Geometry check sheet. Reference: the model listing, model coordinates, mm. A direction names the side the tool comes from. Coordinates: 2 decimals unless noted, no trailing zeros. Loops run counter-clockwise (first coordinate to the right, second up) from the corner with the lowest first, then second, coordinate; pieces in that order, holes last.
from build123d import *

# Parameters (mm, degrees)
F0_W          = 90
F0_H          = 32
F1_DEPTH      = 65.2
F3_DEPTH      = 25
F4_W          = 90
F4_H          = 65.2
F5_DEPTH      = 32.001
F6_DEPTH      = 62.5
F8_DEPTH      = 16.25
F8_DEPTH_BACK = 78.75
F9_R          = 2
F11_DEPTH     = 78.751


with BuildPart() as f1:
    # F0 (on Front) → F1 (new body)
    with BuildSketch(Plane.XZ):
        with Locations((-2.4301670492, -5.0586230417)):
            Rectangle(F0_W, F0_H)
    extrude(amount=F1_DEPTH)

    # F2 (on face) → F3 (join)
    with BuildSketch(Plane.XZ.offset(65.2)):
        with BuildLine():
            Line((40.5698329508, 10.9413769583), (-45.4301670492, 10.9413769583))
            ThreePointArc((-45.4301670492, 10.9413769583), (-46.8443806115, 10.3555905207), (-47.4301670492, 8.9413769583))
            Line((-47.4301670492, 8.9413769583), (-47.4301670492, 2.9413769583))
            ThreePointArc((-47.4301670492, 2.9413769583), (-46.8443806115, 1.5271633959), (-45.4301670492, 0.9413769583))
            Line((-45.4301670492, 0.9413769583), (-42.2728696535, 0.9413769583))
            ThreePointArc((-42.2728696535, 0.9413769583), (-41.1580897163, 0.6018785968), (-40.4217757411, -0.3013573503))
            Line((-40.4217757411, -0.3013573503), (-32.4385583572, -19.8158887331))
            ThreePointArc((-32.4385583572, -19.8158887331), (-31.7022443821, -20.7191246802), (-30.5874644448, -21.0586230417))
            Line((-30.5874644448, -21.0586230417), (25.7271303465, -21.0586230417))
            ThreePointArc((25.7271303465, -21.0586230417), (26.8419102837, -20.7191246802), (27.5782242589, -19.8158887331))
            Line((27.5782242589, -19.8158887331), (35.5614416428, -0.3013573503))
            ThreePointArc((35.5614416428, -0.3013573503), (36.2977556179, 0.6018785968), (37.4125355552, 0.9413769583))
            Line((37.4125355552, 0.9413769583), (40.5698329508, 0.9413769583))
            ThreePointArc((40.5698329508, 0.9413769583), (41.9840465132, 1.5271633959), (42.5698329508, 2.9413769583))
            Line((42.5698329508, 2.9413769583), (42.5698329508, 8.9413769583))
            ThreePointArc((42.5698329508, 8.9413769583), (41.9840465132, 10.3555905207), (40.5698329508, 10.9413769583))
        make_face()
    extrude(amount=F3_DEPTH)

    # F4 (on face) → F5 (cut, through all)
    with BuildSketch(Plane.XY.offset(10.9413769583)):
        with Locations((-2.4301670492, -32.6)):
            Rectangle(F4_W, F4_H)
    extrude(amount=-F5_DEPTH, mode=Mode.SUBTRACT)

    # F6 (add): a face of the model
    f6_faces = [f1.faces().sort_by_distance(p)[0] for p in [
        (-2.4301670492, -90.2, -3.7537517767),
    ]]
    extrude(f6_faces, amount=-F6_DEPTH)

    # F7 (on face) → F8 (join, two sides)
    with BuildSketch(Plane.XZ.offset(90.2)) as f8_sk:
        with BuildLine():
            Line((21.5698329508, 10.9413769583), (-26.4301670492, 10.9413769583))
            ThreePointArc((-26.4301670492, 10.9413769583), (-27.8443806115, 10.3555905207), (-28.4301670492, 8.9413769583))
            Line((-28.4301670492, 8.9413769583), (-28.4301670492, -19.0586230417))
            ThreePointArc((-28.4301670492, -19.0586230417), (-27.8443806115, -20.4728366041), (-26.4301670492, -21.0586230417))
            Line((-26.4301670492, -21.0586230417), (-16.4301670492, -21.0586230417))
            Line((-16.4301670492, -21.0586230417), (-16.4301670492, -9.1799433853))
            Line((-16.4301670492, -9.1799433853), (-14.3088467056, -7.0586230417))
            Line((-14.3088467056, -7.0586230417), (9.4485126073, -7.0586230417))
            Line((9.4485126073, -7.0586230417), (11.5698329508, -9.1799433853))
            Line((11.5698329508, -9.1799433853), (11.5698329508, -21.0586230417))
            Line((11.5698329508, -21.0586230417), (21.5698329508, -21.0586230417))
            ThreePointArc((21.5698329508, -21.0586230417), (22.9840465132, -20.4728366041), (23.5698329508, -19.0586230417))
            Line((23.5698329508, -19.0586230417), (23.5698329508, 8.9413769583))
            ThreePointArc((23.5698329508, 8.9413769583), (22.9840465132, 10.3555905207), (21.5698329508, 10.9413769583))
        make_face()
    extrude(amount=F8_DEPTH)
    extrude(f8_sk.sketch, amount=-F8_DEPTH_BACK)

    # F9
    f9_edges = [f1.edges().sort_by_distance(p)[0] for p in [
        (-28.430167, -106.45, -5.058623),
        (-2.430167, -11.45, 10.941377),
    ]]
    fillet(f9_edges, radius=F9_R)

    # F10 (on face) → F11 (cut, through all)
    with BuildSketch(Plane.XZ.offset(90.2)):
        Polygon((-16.4301670492, -9.1799433853), (-16.4301670492, -21.0586230417), (11.5698329508, -21.0586230417), (11.5698329508, -9.1799433853), (9.4485126073, -7.0586230417), (-14.3088467056, -7.0586230417), align=None)
    extrude(amount=-F11_DEPTH, mode=Mode.SUBTRACT)


solid = f1.part
(1) Gauge pin test, flat ends, axial feed: pin 1 Ø5 at (x, z) = (-38, 3.5) entering from +Y; pin 2 Ø7 at (y, z) = (-22, 0.5) entering from -X; pin 3 Ø4.5 at (y, z) = (-20, -10) entering from +X. Record the tip position at first contact, or that the pin passes through.
Findings:
pin 1: stops at y = -27.7
pin 2: stops at x = -28.43
pin 3: stops at x = 23.57
(2) Sectioned sample at A-A on x = -12.5. Record the cut outline in (y, z), and give its area (3 significant figures).
Findings:
outline: (-106.45, -7.06) - (-11.45, -7.06) - (-11.45, 8.94) arc R2 ccw to (-13.45, 10.94) - (-104.45, 10.94) arc R2 ccw to (-106.45, 8.94) - close
area: 1,710 mm2
(3) Sectioned sample at B-B on y = -36. Record the cut outline in (x, z).
Findings:
outline: (-47.43, 2.94) arc R2 ccw to (-45.43, 0.94) - (-42.27, 0.94) arc R2 cw to (-40.42, -0.3) - (-32.44, -19.82) arc R2 ccw to (-30.59, -21.06) - (-16.43, -21.06) - (-16.43, -9.18) - (-14.31, -7.06) - (9.45, -7.06) - (11.57, -9.18) - (11.57, -21.06) - (25.73, -21.06) arc R2 ccw to (27.58, -19.82) - (35.56, -0.3) arc R2 cw to (37.41, 0.94) - (40.57, 0.94) arc R2 ccw to (42.57, 2.94) - (42.57, 8.94) arc R2 ccw to (40.57, 10.94) - (-45.43, 10.94) arc R2 ccw to (-47.43, 8.94) - close
(4) Draft check along X on faces 1 (the flat face through (-47.43, -59, 6)), 2 (the flat face through (39, -59, 0.941)), 3 (the flat face through (-16.43, -60, -15)), 4 (the flat face through (-3, -60, -7.059)). Enter one of: +X half, -X half, draft (parallel to the pull), parting line (faces both ways), or undercut.
Findings:
face 1: -X half
face 2: draft
face 3: undercut
face 4: undercut
(5) Scan lines: L1, parallel to X at y = -18.5, z = -17; L2, parallel to Z at x = 31, y = -61; L3, parallel to Z at x = -12, y = -79.5. Record each from-to range of solid material in increasing order.
Findings:
L1: x = -28.43 to -16.43, 11.57 to 23.57
L2: z = -11.45 to 10.94
L3: z = -7.06 to 10.94
(6) Sectioned sample at D-D on z = 5.5. Record the cut outline in (x, y).
Findings:
outline: (-47.43, -90.2) - (-28.43, -90.2) - (-28.43, -104.45) arc R2 ccw to (-26.43, -106.45) - (21.57, -106.45) arc R2 ccw to (23.57, -104.45) - (23.57, -90.2) - (42.57, -90.2) - (42.57, -27.7) - (23.57, -27.7) - (23.57, -13.45) arc R2 ccw to (21.57, -11.45) - (-26.43, -11.45) arc R2 ccw to (-28.43, -13.45) - (-28.43, -27.7) - (-47.43, -27.7) - close
(7) Sectioned sample at C-C on z = -16.5. Record the cut outline in (x, y).
Findings:
outline: (-33.8, -90.2) - (-28.43, -90.2) - (-28.43, -104.45) arc R2 ccw to (-26.43, -106.45) - (-16.43, -106.45) - (-16.43, -11.45) - (-26.43, -11.45) arc R2 ccw to (-28.43, -13.45) - (-28.43, -27.7) - (-33.8, -27.7) - close; (11.57, -106.45) - (21.57, -106.45) arc R2 ccw to (23.57, -104.45) - (23.57, -90.2) - (28.93, -90.2) - (28.93, -27.7) - (23.57, -27.7) - (23.57, -13.45) arc R2 ccw to (21.57, -11.45) - (11.57, -11.45) - close
(8) Access from +Z, -Z, +X, -X, +Y, -Y to the whole of each face (thin tool, end or side, straight path). Record for faces 5 (the flat face through (-28.43, -97, -5)), 6 (the flat face through (23.57, -97, -5)), 7 (the flat face through (-15.38, -59.62, -8.13)), 8 (the flat face through (23.57, -21, -5)).
Findings:
face 5: +Z, -Z, -X, -Y
face 6: +Z, -Z, +X, -Y
face 7: -Z, +Y, -Y
face 8: +Z, -Z, +X, +Y
